from build123d import *

# Parameters (mm, degrees)
F0_W         = 38.7927275151
F0_H         = 10.5539034121
F1_DEPTH     = 25.4
F2_W         = 8.5572190583
F2_H         = 29.094544705
F3_DEPTH     = 20.32
F4_W         = 8.5572199896
F4_H         = 28.5240663216
F5_DEPTH     = 17.78
F6_R         = 5.4792946357
F7_DEPTH     = 27.94
F8_W         = 23.1044916436
F8_H         = 6.5605361015
F9_DEPTH     = 25.4
F10_T1_DEPTH = 64.1927275151
F10_T3_DEPTH = 38.1
F10_T5_DEPTH = 48.5044916436
F10_T7_DEPTH = 50.8


# Not quite as in the source:
# - a fillet or chamfer that OpenCascade refuses, or shapes differently, is made with other operations: its cross-section is extruded or revolved along the edge and cut away or added


with BuildPart() as f1:
    # F0 (on Front) → F1 (new body)
    with BuildSketch(Plane.XZ):
        with Locations((0.2852408215, -0.2852405887)):
            Rectangle(F0_W, F0_H)
    extrude(amount=F1_DEPTH)

    # F2 (on Right) → F3 (join)
    with BuildSketch(Plane.YZ):
        with Locations((4.2786095291, 10.1260424126)):
            Rectangle(F2_W, F2_H)
    extrude(amount=F3_DEPTH)

    # F4 (on Right) → F5 (join)
    with BuildSketch(Plane.YZ):
        with Locations((4.2786099948, 10.1260435767)):
            Rectangle(F4_W, F4_H)
    extrude(amount=-F5_DEPTH)

    # F6 (on Top) → F7 (join)
    with BuildSketch(Plane.XY):
        with Locations((0, -12.9784494638)):
            Circle(F6_R)
    extrude(amount=-F7_DEPTH)

    # F8 (on Front) → F9 (join)
    with BuildSketch(Plane.XZ):
        with Locations((-0.1426204108, -31.0912309214)):
            Rectangle(F8_W, F8_H)
    extrude(amount=F9_DEPTH)

    # F10: fillet of radius 5.08 on 7 edges, made by hand

    # F10_s2 → F10_t1 (cut)
    with BuildSketch(Plane.YZ.offset(-31.811122936)):
        with BuildLine():
            ThreePointArc((-20.32, 4.9917111173), (-23.9121024484, 3.5038135658), (-25.4, -0.0882888827))
            Line((-25.4, -0.0882888827), (-25.4, 4.9917111173))
            Line((-25.4, 4.9917111173), (-20.32, 4.9917111173))
        make_face()
    extrude(amount=F10_T1_DEPTH, mode=Mode.SUBTRACT)

    # F10_s4 → F10_t3 (cut)
    with BuildSketch(Plane.XZ):
        with BuildLine():
            ThreePointArc((-14.031122936, 4.9917111173), (-17.6232253844, 3.5038135658), (-19.111122936, -0.0882888827))
            Line((-19.111122936, -0.0882888827), (-19.111122936, 4.9917111173))
            Line((-19.111122936, 4.9917111173), (-14.031122936, 4.9917111173))
        make_face()
        with BuildLine():
            ThreePointArc((14.6016045791, 4.9917111173), (18.1937070275, 3.5038135658), (19.6816045791, -0.0882888827))
            Line((19.6816045791, -0.0882888827), (19.6816045791, 4.9917111173))
            Line((19.6816045791, 4.9917111173), (14.6016045791, 4.9917111173))
        make_face()
    extrude(amount=F10_T3_DEPTH, mode=Mode.SUBTRACT)

    # F10_s6 → F10_t5 (cut)
    with BuildSketch(Plane.YZ.offset(-24.3948662326)):
        with BuildLine():
            ThreePointArc((-20.32, -27.8109628707), (-23.9121024484, -29.2988604223), (-25.4, -32.8909628707))
            Line((-25.4, -32.8909628707), (-25.4, -27.8109628707))
            Line((-25.4, -27.8109628707), (-20.32, -27.8109628707))
        make_face()
        with BuildLine():
            ThreePointArc((-5.08, -27.8109628707), (-1.4878975516, -29.2988604223), (0, -32.8909628707))
            Line((0, -32.8909628707), (0, -27.8109628707))
            Line((0, -27.8109628707), (-5.08, -27.8109628707))
        make_face()
    extrude(amount=F10_T5_DEPTH, mode=Mode.SUBTRACT)

    # F10_s8 → F10_t7 (cut)
    with BuildSketch(Plane.XZ.offset(-12.7)):
        with BuildLine():
            ThreePointArc((6.329625411, -27.8109628707), (9.9217278595, -29.2988604223), (11.409625411, -32.8909628707))
            Line((11.409625411, -32.8909628707), (11.409625411, -27.8109628707))
            Line((11.409625411, -27.8109628707), (6.329625411, -27.8109628707))
        make_face()
        with BuildLine():
            ThreePointArc((-6.6148662326, -27.8109628707), (-10.206968681, -29.2988604223), (-11.6948662326, -32.8909628707))
            Line((-11.6948662326, -32.8909628707), (-11.6948662326, -27.8109628707))
            Line((-11.6948662326, -27.8109628707), (-6.6148662326, -27.8109628707))
        make_face()
    extrude(amount=F10_T7_DEPTH, mode=Mode.SUBTRACT)


solid = f1.part
Geometry: final body of the model. Coordinates: model frame, mm. A direction names the side the tool comes from. Coordinates: 2 decimals unless noted, no trailing zeros. Write each loop counter-clockwise with the first axis right and the second up, starting at its lowest first coordinate (ties: lowest second). Pieces come first, ordered by that corner, then holes. Notation, with made-up numbers: (56.5, 79.5) - (67.5, 79.5) arc R31 ccw to (67.5, 114.5) - close; hole circle Ø5 at (39, 89). An arc over 180 degrees is marked (long way). Return JSON: item names as keys, results as strings.
Item 1: Section query C-C (y = 1). Output: boundary loops of the cut face in (x, z).
Completed:
{"outline": "(-17.78, -4.14) - (0, -4.14) - (0, -4.42) - (20.32, -4.42) - (20.32, 24.67) - (0, 24.67) - (0, 24.39) - (-17.78, 24.39) - close"}
Item 2: Section query A-A (y = -21). Output: boundary loops of the cut face in (x, z), and give its area (3 significant figures).
Completed:
{"outline": "(-19.11, -5.56) - (19.68, -5.56) - (19.68, -0.09) arc R5.08 ccw to (15.28, 4.95) - (-14.71, 4.95) arc R5.08 ccw to (-19.11, -0.09) - close; (-11.69, -34.37) - (11.41, -34.37) - (11.41, -32.89) arc R5.08 ccw to (7.01, -27.86) - (-7.29, -27.86) arc R5.08 ccw to (-11.69, -32.89) - close", "area": "537 mm2"}
Item 3: Reachability of faces 1 (the face through (-9, 4, 24.388)), 2 (the face through (-10.17, -12.52, -29.26)), 3 (the face through (19.682, -13, -3)), 4 (the face through (-0.3, -23.87, -29.26)) from +Z, -Z, +X, -X, +Y, -Y: full face, straight path, thin tool, end or side. Return the list, or none.
Completed:
{"face 1": "+Z, -X, +Y, -Y", "face 2": "-X, +Y, -Y", "face 3": "+Z, -Z, +X, -Y", "face 4": "+X, -X, -Y"}
Item 4: Section query B-B (x = -15.5). Output: boundary loops of the cut face in (y, z), and give its area (3 significant figures).
Completed:
{"outline": "(-25.4, -5.56) - (0, -5.56) - (0, -4.14) - (8.56, -4.14) - (8.56, 24.39) - (0, 24.39) - (0, 4.77) - (-21.79, 4.77) arc R5.08 ccw to (-25.4, -0.09) - close", "area": "502 mm2"}
Item 5: Pin query (flat end, axial travel): pin 1 Ø1.6 at (y, z) = (-17, -1.5) entering from +X; pin 2 Ø7 at (x, y) = (9.5, 4.5) entering from -Z; pin 3 Ø7 at (x, y) = (-7.5, 3) entering from +Z. Return the tip coordinate at first contact, or that it passes through.
Completed:
{"pin 1": "stops at x = 19.68", "pin 2": "stops at z = -4.42", "pin 3": "stops at z = 24.39"}
Item 6: Line query: L1, parallel to X at y = -17, z = -5; L2, parallel to Z at x = 18, y = 7; L3, parallel to Z at x = 1, y = -6. Output: solid intervals per line, ascending.
Completed:
{"L1": "x = -19.11 to 19.68", "L2": "z = -4.42 to 24.67", "L3": "z = -34.37 to -27.81, -5.56 to 4.99"}
